Read the model definition and answer for the solid it produces. Units are mm, in the model's axes. Face numbers are marked on the shaded views. A direction names the side the tool comes from. Round coordinates to 2 decimals unless told otherwise and drop trailing zeros. Order: outer loops, then holes, each group sorted by start corner. A loop starts at its lowest first (then second) coordinate and runs counter-clockwise, first axis right, second up. Notation, with made-up numbers: (-26, 18.25) -> (-12, 18.25) arc R22 cw to (-12, 26.25) -> close; hole circle Ø7 at (-18, -12.75). An arc over 180 degrees is marked (long way). One line per item, written item: value. Start each with the question number.
1. Section B-B (z = 7.5) is taken. Give the vertices of the cut face in (x, y), then the cut area to 3 significant figures.
2. Section C-C (x = -12) is taken. Give the vertices of the cut face in (y, z).
3. Consider line 1 (Y direction, x = 12, z = 1.3); line 2 (Y direction, x = -2, z = 3.25); line 3 (Z direction, x = -6.5, y = -16). Determine where each line is inside the solid, lowest interval first.
4. The mould has two halves that part along X. Classify the marked faces 4, 5 and 6: released by +X, released by -X, zero draft, split by the parting line, or undercut.
5. Section A-A (y = 17) is taken. Give the vertices of the cut face in (x, z).
6. Section D-D (z = 2.25) is taken. Give the vertices of the cut face in (x, y).
7. Flat-ended cylindrical pins translate along their axes: pin 1 Ø5 at (y, z) = (17.5, 6.5) entering from +X; pin 2 Ø17 at (x, y) = (4, -3.5) entering from +Z; pin 3 Ø5.5 at (x, z) = (-9.5, 5.5) entering from +Y; pin 4 Ø1 at (y, z) = (-11, 3.5) entering from -X. Find the tip coordinate at first contact, or state that the pin passes through.
8. For the marked faces 1, 2 and 3, determine the directions among +Z, -Z, +X, -X, +Y, -Y from which every point of the face is accessible in a straight line to the end or side of a thin tool.
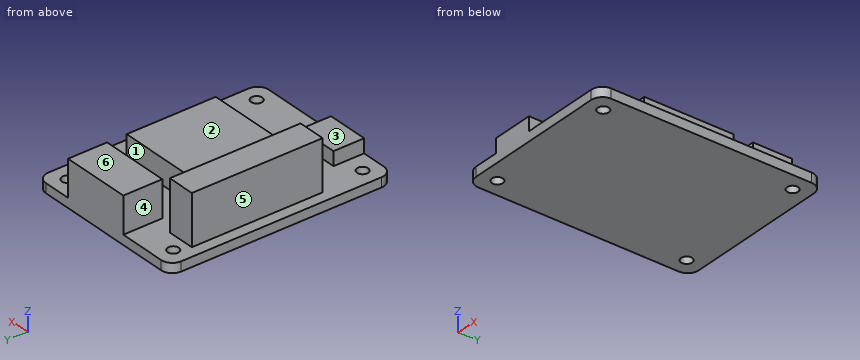
from build123d import *

# Parameters (mm, degrees)
SKETCH_1_W      = 30.1
SKETCH_1_H      = 40
SKETCH_1_R      = 1
EXTRUDE_1_DEPTH = 1.7
SKETCH_2_W      = 5
SKETCH_2_H      = 23.5
EXTRUDE_2_DEPTH = 9
SKETCH_3_W      = 15.5
SKETCH_3_H      = 16
EXTRUDE_3_DEPTH = 4.5
SKETCH_4_W      = 12.5
SKETCH_4_H      = 7
EXTRUDE_4_DEPTH = 6.5
SKETCH_5_W      = 7.5
SKETCH_5_H      = 5.5
EXTRUDE_5_DEPTH = 2.5
FILLET_1_R      = 2


with BuildPart() as part:
    # 草图1 → 凸台-拉伸1 (new body)
    with BuildSketch(Plane.XY):
        Rectangle(SKETCH_1_W, SKETCH_1_H)
        with Locations((12, 17)):
            Circle(SKETCH_1_R, mode=Mode.SUBTRACT)
        with Locations((-12, 17)):
            Circle(SKETCH_1_R, mode=Mode.SUBTRACT)
        with Locations((-12, -17)):
            Circle(SKETCH_1_R, mode=Mode.SUBTRACT)
        with Locations((12, -17)):
            Circle(SKETCH_1_R, mode=Mode.SUBTRACT)
    extrude(amount=EXTRUDE_1_DEPTH)

    # 草图2 → 凸台-拉伸2 (add)
    with BuildSketch(Plane.XY.offset(1.7)):
        with Locations((-10.55, 2.75)):
            Rectangle(SKETCH_2_W, SKETCH_2_H)
    extrude(amount=EXTRUDE_2_DEPTH)

    # 草图3 → 凸台-拉伸3 (add)
    with BuildSketch(Plane.XY.offset(1.7)):
        with Locations((2.8, -0.5)):
            Rectangle(SKETCH_3_W, SKETCH_3_H)
    extrude(amount=EXTRUDE_3_DEPTH)

    # 草图4 → 凸台-拉伸4 (add)
    with BuildSketch(Plane.XY.offset(1.7)):
        with Locations((1.8, 16.5)):
            Rectangle(SKETCH_4_W, SKETCH_4_H)
    extrude(amount=EXTRUDE_4_DEPTH)

    # 草图5 → 凸台-拉伸5 (add)
    with BuildSketch(Plane.XY.offset(1.7)):
        with Locations((-4.8, -17.25)):
            Rectangle(SKETCH_5_W, SKETCH_5_H)
    extrude(amount=EXTRUDE_5_DEPTH)

    # 圆角1
    fillet_1_edges = [part.edges().sort_by_distance(p)[0] for p in [
        (-15.05, 20, 0.85),
        (15.05, 20, 0.85),
        (15.05, -20, 0.85),
        (-15.05, -20, 0.85),
    ]]
    fillet(fillet_1_edges, radius=FILLET_1_R)


solid = part.part
Answer:
1. outline: (-13.05, -9) -> (-8.05, -9) -> (-8.05, 14.5) -> (-13.05, 14.5) -> close; (-4.45, 13) -> (8.05, 13) -> (8.05, 20) -> (-4.45, 20) -> close
1. area: 205 mm^2
2. outline: (-20, 0) -> (-18, 0) -> (-18, 1.7) -> (-20, 1.7) -> close; (-16, 0) -> (16, 0) -> (16, 1.7) -> (14.5, 1.7) -> (14.5, 10.7) -> (-9, 10.7) -> (-9, 1.7) -> (-16, 1.7) -> close; (18, 0) -> (20, 0) -> (20, 1.7) -> (18, 1.7) -> close
3. line 1: -20 to -18, -16 to 16, 18 to 20
3. line 2: -20 to -14.5, -8.5 to 7.5, 13 to 20
3. line 3: 0 to 4.2
4. face 4: undercut
4. face 5: released by -X
4. face 6: zero draft
5. outline: (-15.05, 0) -> (-13, 0) -> (-13, 1.7) -> (-15.05, 1.7) -> close; (-11, 0) -> (11, 0) -> (11, 1.7) -> (8.05, 1.7) -> (8.05, 8.2) -> (-4.45, 8.2) -> (-4.45, 1.7) -> (-11, 1.7) -> close; (13, 0) -> (15.05, 0) -> (15.05, 1.7) -> (13, 1.7) -> close
6. outline: (-13.05, -9) -> (-8.05, -9) -> (-8.05, 14.5) -> (-13.05, 14.5) -> close; (-8.55, -20) -> (-1.05, -20) -> (-1.05, -14.5) -> (-8.55, -14.5) -> close; (-4.95, -8.5) -> (10.55, -8.5) -> (10.55, 7.5) -> (-4.95, 7.5) -> close; (-4.45, 13) -> (8.05, 13) -> (8.05, 20) -> (-4.45, 20) -> close
7. pin 1: x = 8.05
7. pin 2: z = 6.2
7. pin 3: y = 14.5
7. pin 4: through
8. face 1: +Z, +X
8. face 2: +Z, +X, -Y
8. face 3: +Z, +X, -X, -Y
